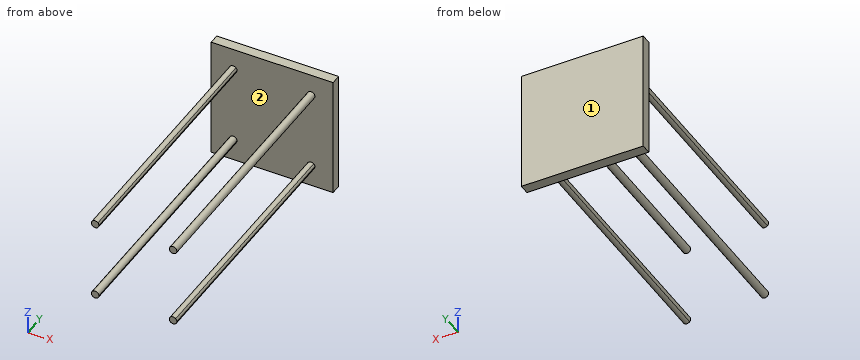
from build123d import *

# Parameters (mm, degrees)
F0_W     = 304.8
F0_H     = 304.8
F1_DEPTH = 25.4
F2_DEPTH = 660.4


with BuildPart() as f1:
    # F0 (on Front) → F1 (new body)
    with BuildSketch(Plane.XZ):
        with Locations((-11.4630328134, -11.4630328134)):
            Rectangle(F0_W, F0_H)
        with BuildLine():
            ThreePointArc((92.4711311021, 79.0087948248), (117.5894180385, 36.8373497331), (126.3319671866, -11.4630328134))
            ThreePointArc((126.3319671866, -11.4630328134), (117.5894180385, -59.7634153598), (92.4711311021, -101.9348604515))
            ThreePointArc((92.4711311021, -101.9348604515), (94.708384089, -105.1022008793), (95.4977461002, -108.898811727))
            ThreePointArc((95.4977461002, -108.898811727), (89.4651656842, -117.7604498627), (79.0087948248, -115.3971967289))
            ThreePointArc((79.0087948248, -115.3971967289), (-11.4630328134, -149.2580328134), (-101.9348604515, -115.3971967289))
            ThreePointArc((-101.9348604515, -115.3971967289), (-115.6340038178, -115.6340038178), (-115.3971967289, -101.9348604515))
            ThreePointArc((-115.3971967289, -101.9348604515), (-149.2580328134, -11.4630328134), (-115.3971967289, 79.0087948248))
            ThreePointArc((-115.3971967289, 79.0087948248), (-115.6340038178, 92.707938191), (-101.9348604515, 92.4711311021))
            ThreePointArc((-101.9348604515, 92.4711311021), (-11.4630328134, 126.3319671866), (79.0087948248, 92.4711311021))
            ThreePointArc((79.0087948248, 92.4711311021), (89.4651656842, 94.834384236), (95.4977461002, 85.9727461002))
            ThreePointArc((95.4977461002, 85.9727461002), (94.708384089, 82.1761352526), (92.4711311021, 79.0087948248))
        make_face(mode=Mode.SUBTRACT)
        with BuildLine():
            ThreePointArc((92.4711311021, -101.9348604515), (117.5894180385, -59.7634153598), (126.3319671866, -11.4630328134))
            ThreePointArc((126.3319671866, -11.4630328134), (117.5894180385, 36.8373497331), (92.4711311021, 79.0087948248))
            ThreePointArc((92.4711311021, 79.0087948248), (79.2375540094, 79.2375540094), (79.0087948248, 92.4711311021))
            ThreePointArc((79.0087948248, 92.4711311021), (-11.4630328134, 126.3319671866), (-101.9348604515, 92.4711311021))
            ThreePointArc((-101.9348604515, 92.4711311021), (-100.0371735912, 89.4651656842), (-99.373811727, 85.9727461002))
            ThreePointArc((-99.373811727, 85.9727461002), (-105.1022008793, 77.2371081114), (-115.3971967289, 79.0087948248))
            ThreePointArc((-115.3971967289, 79.0087948248), (-149.2580328134, -11.4630328134), (-115.3971967289, -101.9348604515))
            ThreePointArc((-115.3971967289, -101.9348604515), (-105.1022008793, -100.1631737382), (-99.373811727, -108.898811727))
            ThreePointArc((-99.373811727, -108.898811727), (-100.0371735912, -112.391231311), (-101.9348604515, -115.3971967289))
            ThreePointArc((-101.9348604515, -115.3971967289), (-11.4630328134, -149.2580328134), (79.0087948248, -115.3971967289))
            ThreePointArc((79.0087948248, -115.3971967289), (79.2375540094, -102.1636196362), (92.4711311021, -101.9348604515))
        make_face()
        with BuildLine():
            ThreePointArc((79.0087948248, 92.4711311021), (79.2375540094, 79.2375540094), (92.4711311021, 79.0087948248))
            ThreePointArc((92.4711311021, 79.0087948248), (85.9727461002, 85.9727461002), (79.0087948248, 92.4711311021))
        make_face()
    extrude(amount=F1_DEPTH)

    # F0 (on Front) → F2 (join)
    with BuildSketch(Plane.XZ):
        with BuildLine():
            ThreePointArc((79.0087948248, 92.4711311021), (79.2375540094, 79.2375540094), (92.4711311021, 79.0087948248))
            ThreePointArc((92.4711311021, 79.0087948248), (85.9727461002, 85.9727461002), (79.0087948248, 92.4711311021))
        make_face()
        with BuildLine():
            ThreePointArc((79.0087948248, 92.4711311021), (85.9727461002, 85.9727461002), (92.4711311021, 79.0087948248))
            ThreePointArc((92.4711311021, 79.0087948248), (94.708384089, 82.1761352526), (95.4977461002, 85.9727461002))
            ThreePointArc((95.4977461002, 85.9727461002), (89.4651656842, 94.834384236), (79.0087948248, 92.4711311021))
        make_face()
        with BuildLine():
            ThreePointArc((95.4977461002, -108.898811727), (94.708384089, -105.1022008793), (92.4711311021, -101.9348604515))
            ThreePointArc((92.4711311021, -101.9348604515), (85.9727461002, -108.898811727), (79.0087948248, -115.3971967289))
            ThreePointArc((79.0087948248, -115.3971967289), (89.4651656842, -117.7604498627), (95.4977461002, -108.898811727))
        make_face()
        with BuildLine():
            ThreePointArc((79.0087948248, -115.3971967289), (85.9727461002, -108.898811727), (92.4711311021, -101.9348604515))
            ThreePointArc((92.4711311021, -101.9348604515), (79.2375540094, -102.1636196362), (79.0087948248, -115.3971967289))
        make_face()
        with BuildLine():
            ThreePointArc((-99.373811727, 85.9727461002), (-100.0371735912, 89.4651656842), (-101.9348604515, 92.4711311021))
            ThreePointArc((-101.9348604515, 92.4711311021), (-108.898811727, 85.9727461002), (-115.3971967289, 79.0087948248))
            ThreePointArc((-115.3971967289, 79.0087948248), (-105.1022008793, 77.2371081114), (-99.373811727, 85.9727461002))
        make_face()
        with BuildLine():
            ThreePointArc((-115.3971967289, 79.0087948248), (-108.898811727, 85.9727461002), (-101.9348604515, 92.4711311021))
            ThreePointArc((-101.9348604515, 92.4711311021), (-115.6340038178, 92.707938191), (-115.3971967289, 79.0087948248))
        make_face()
        with BuildLine():
            ThreePointArc((-115.3971967289, -101.9348604515), (-115.6340038178, -115.6340038178), (-101.9348604515, -115.3971967289))
            ThreePointArc((-101.9348604515, -115.3971967289), (-108.898811727, -108.898811727), (-115.3971967289, -101.9348604515))
        make_face()
        with BuildLine():
            ThreePointArc((-115.3971967289, -101.9348604515), (-108.898811727, -108.898811727), (-101.9348604515, -115.3971967289))
            ThreePointArc((-101.9348604515, -115.3971967289), (-100.0371735912, -112.391231311), (-99.373811727, -108.898811727))
            ThreePointArc((-99.373811727, -108.898811727), (-105.1022008793, -100.1631737382), (-115.3971967289, -101.9348604515))
        make_face()
    extrude(amount=F2_DEPTH)


solid = f1.part
Verification items for the finished model (mm, model axes). Face numbers are marked on the shaded views. A direction names the side the tool comes from. Give positions to 0.01 mm unless a question says otherwise; leave off trailing zeros. Write each loop counter-clockwise with the first axis right and the second up, starting at its lowest first coordinate (ties: lowest second). Pieces come first, ordered by that corner, then holes. Notation, with made-up numbers: M -5.5,40.5 L 42.5,40.5 A19 cw 42.5,68.5 Z; hole C 57.5,1 d9. An arc over 180 degrees is marked long. Use CSV: the item, a comma, the result in double quotes.
1) Cross-section at A-A (y = -321.5). Enter the section's corners in (x, z) (3 decimals).
Final values:
outline,"C -108.899,-108.899 d19.05; C -108.899,85.973 d19.05; C 85.973,-108.899 d19.05; C 85.973,85.973 d19.05"
2) Cross-section at B-B (x = 55). Enter the section's corners in (y, z), plus the area to 3 significant figures.
Final values:
outline,"M -25.4,-163.86 L 0,-163.86 L 0,140.94 L -25.4,140.94 Z"
area,"7,740 mm²"
3) Cross-section at C-C (z = -27.5). Enter the section's corners in (x, y).
Final values:
outline,"M -163.86,-25.4 L 140.94,-25.4 L 140.94,0 L -163.86,0 Z"
4) Go/stop test with flat-tipped pins: pin 1 Ø3 at (x, z) = (27.5, 64.5) entering from -Y; pin 2 Ø10 at (y, z) = (-168.5, -96) entering from -X. Record where each tip stops, or that it passes through.
Final values:
pin 1,"y = -25.4"
pin 2,"x = -114.22"
5) Access from +Z, -Z, +X, -X, +Y, -Y to the whole of each face (thin tool, end or side, straight path). Record for the marked faces 1 and 2.
Final values:
face 1,"+Z, -Z, +X, -X, +Y"
face 2,"-Y"
6) Material ranges on line 1 along Y through (x, z) = (-110.5, -23.5); line 2 along X through (y, z) = (-342, 82); line 3 along Z through (x, y) = (82.5, -290), recorded low to high.
Final values:
line 1,"-25.4 to 0"
line 2,"-117.56 to -100.24, 77.32 to 94.63"
line 3,"-117.77 to -100.03, 77.1 to 94.84"
